Work out the finished part from the listing and answer in its coordinate system (mm). A direction names the side the tool comes from. Give positions to 0.01 mm unless a question says otherwise; leave off trailing zeros. Order: outer loops, then holes, each group sorted by start corner. A loop starts at its lowest first (then second) coordinate and runs counter-clockwise, first axis right, second up. Notation, with made-up numbers: (65.25, 1.5) -> (113.25, 1.5) arc R19 cw to (113.25, 37.5) -> close; hole circle Ø9 at (83.5, 48). An arc over 180 degrees is marked (long way). Answer as CSV lines item,"result". Start each with the question number.
1. Find the intervals of material crossed by L1, parallel to X at y = 76, z = 3.45, in increasing order.
2. A cutting plane is placed at B-B (y = 47.5). Give the vertices of the cut face in (x, z).
3. A cutting plane is placed at A-A (x = 12). Give the vertices of the cut face in (y, z).
4. For faces 4 (the flat face through (-5, 11, 3)), 5 (the flat face through (9, 79, 2)), 6 (the flat face through (0, 49, 2)), determine the directions among +Z, -Z, +X, -X, +Y, -Y from which every point of the face is accessible in a straight line to the end or side of a thin tool.
5. For a pull along X with two mould halves and no side action, classify faces 1 (the flat face through (4, 0, 3)), 2 (the flat face through (11, 45.273, 3)), 3 (the flat face through (-5, 26, 3)) as released by +X, released by -X, zero draft, split by the parting line, or undercut.
6. Flat-ended cylindrical pins translate along their axes: pin 1 (1 mm diameter, centred on y = 33, z = 3, fed in from +X); pin 2 (1.2 mm diameter, centred on x = 4, z = 2.5, fed in from +Y). Find the tip coordinate at first contact, or state that the pin passes through.
Autodesk Fusion 360 part; units mm, degrees
sketch "Sketch1" plane through (0, 0, 0) normal (0, 0, 1) x (1, 0, 0)
  line L0 (0, 0) -> (9, 0)
  line L1 (9, 0) -> (9, 83)
  line L2 (9, 83) -> (0, 83)
  line L3 (0, 83) -> (0, 0)
  dimension "d5" = 9
  dimension "d6" = 83
extrude "Extrude1" add sketch "Sketch1" along normal blind 5
sketch "Sketch2" plane through (9, 0, 0) normal (1, 0, 0) x (0, 1, 0)
  line L0 (0, 0) -> (83, 0)
  line L1 (83, 0) -> (83, 5)
  line L2 (83, 5) -> (0, 5)
  line L3 (0, 5) -> (0, 0)
  line L4 (7.5455, 5) -> (15.0909, 5)
  line L5 (15.0909, 5) -> (15.0909, 0)
  line L6 (15.0909, 0) -> (7.5455, 0)
  line L7 (7.5455, 0) -> (7.5455, 5)
  line L8 (22.6364, 0) -> (22.6364, 5)
  line L9 (22.6364, 5) -> (30.1818, 5)
  line L10 (30.1818, 0) -> (22.6364, 0)
  line L11 (30.1818, 5) -> (30.1818, 0)
  line L12 (37.7273, 0) -> (37.7273, 5)
  line L13 (37.7273, 5) -> (45.2727, 5)
  line L14 (45.2727, 0) -> (37.7273, 0)
  line L15 (45.2727, 5) -> (45.2727, 0)
  line L16 (52.8182, 0) -> (52.8182, 5)
  line L17 (52.8182, 5) -> (60.3636, 5)
  line L18 (60.3636, 0) -> (52.8182, 0)
  line L19 (60.3636, 5) -> (60.3636, 0)
  line L20 (67.9091, 0) -> (67.9091, 5)
  line L21 (67.9091, 5) -> (75.4545, 5)
  line L22 (75.4545, 0) -> (67.9091, 0)
  line L23 (75.4545, 5) -> (75.4545, 0)
  dimension "d9" = 7.5455
  dimension "d10" = 7.5455
  dimension "d13" = 60.3636
  dimension "d14" = 0
extrude "Extrude2" add sketch "Sketch2" along normal blind 5 contours L0 L2 L4 L5 L6 L7 | L0 L2 L8 L9 L10 L11 | L0 L2 L12 L13 L14 L15 | L0 L2 L16 L17 L18 L19 | L0 L2 L20 L21 L22 L23
sketch "Sketch3" plane through (0, 0, 0) normal (-1, 0, 0) x (0, -1, 0)
  line L0 (-83, 0) -> (0, 0)
  line L1 (0, 0) -> (0, 5)
  line L2 (0, 5) -> (-83, 5)
  line L3 (-83, 5) -> (-83, 0)
  line L4 (-75.4545, 5) -> (-67.9091, 5)
  line L5 (-67.9091, 5) -> (-67.9091, 0)
  line L6 (-67.9091, 0) -> (-75.4545, 0)
  line L7 (-75.4545, 0) -> (-75.4545, 5)
  line L8 (-60.3636, 0) -> (-60.3636, 5)
  line L9 (-60.3636, 5) -> (-52.8182, 5)
  line L10 (-52.8182, 0) -> (-60.3636, 0)
  line L11 (-52.8182, 5) -> (-52.8182, 0)
  line L12 (-45.2727, 0) -> (-45.2727, 5)
  line L13 (-45.2727, 5) -> (-37.7273, 5)
  line L14 (-37.7273, 0) -> (-45.2727, 0)
  line L15 (-37.7273, 5) -> (-37.7273, 0)
  line L16 (-30.1818, 0) -> (-30.1818, 5)
  line L17 (-30.1818, 5) -> (-22.6364, 5)
  line L18 (-22.6364, 0) -> (-30.1818, 0)
  line L19 (-22.6364, 5) -> (-22.6364, 0)
  line L20 (-15.0909, 0) -> (-15.0909, 5)
  line L21 (-15.0909, 5) -> (-7.5455, 5)
  line L22 (-7.5455, 0) -> (-15.0909, 0)
  line L23 (-7.5455, 5) -> (-7.5455, 0)
  point P0 (-75.4545, 5)
  dimension "d17" = 7.5455
  dimension "d20" = 60.3636
  dimension "d21" = 0
extrude "Extrude3" add sketch "Sketch3" along normal blind 5 contours L0 L2 L4 L5 L6 L7 | L0 L2 L8 L9 L10 L11 | L0 L2 L12 L13 L14 L15 | L0 L2 L16 L17 L18 L19 | L0 L2 L20 L21 L22 L23
sketch "Sketch4" plane through (0, 0, 0) normal (0, -1, 0) x (1, 0, 0)
  line L0 (0, 0) -> (9, 0)
  line L1 (9, 0) -> (9, 5)
  line L2 (9, 5) -> (0, 5)
  line L3 (0, 5) -> (0, 0)
sketch "Sketch5" plane through (0, 0, 0) normal (0, 0, 1) x (1, 0, 0)
  line L0 (-5, 0) -> (14, 0)
  line L1 (14, 0) -> (14, -5)
  line L2 (14, -5) -> (-5, -5)
  line L3 (-5, -5) -> (-5, 0)
  line L4 (0, 7.5455) -> (0, 0) construction
  line L5 (0, 0) -> (9, 0)
  point P0 (-5, 7.5455)
  dimension "d24" = 5
  dimension "d25" = 19
  dimension "d44" = 5
extrude "Extrude4" cut sketch "Sketch5" along normal blind 5
extrude "Extrude5" add sketch "Sketch5" along normal blind 5
sketch "Sketch6" plane through (0, 0, 0) normal (0, 0, 1) x (1, 0, 0)
  line L0 (-5, 83) -> (14, 83)
  line L1 (14, 83) -> (14, 88)
  line L2 (14, 88) -> (-5, 88)
  line L3 (-5, 88) -> (-5, 83)
  line L4 (9, 83) -> (0, 83)
  point P0 (0, 83)
  point P1 (-5, 75.4545)
  dimension "d31" = 19
  dimension "d32" = 5
  dimension "d43" = 5
extrude "Extrude6" cut sketch "Sketch6" along normal blind 5
extrude "Extrude7" add sketch "Sketch6" along normal blind 5
sketch "Sketch7" plane through (0, 0, 5) normal (0, 0, 1) x (-1, 0, 0)
  line L0 (0, -83) -> (0, -75.4545)
  line L1 (0, -75.4545) -> (5, -75.4545)
  line L2 (5, -75.4545) -> (5, -67.9091)
  line L3 (5, -67.9091) -> (0, -67.9091)
  line L4 (0, -67.9091) -> (0, -60.3636)
  line L5 (0, -60.3636) -> (5, -60.3636)
  line L6 (5, -60.3636) -> (5, -52.8182)
  line L7 (5, -52.8182) -> (0, -52.8182)
  line L8 (0, -52.8182) -> (0, -45.2727)
  line L9 (0, -45.2727) -> (5, -45.2727)
  line L10 (5, -45.2727) -> (5, -37.7273)
  line L11 (5, -37.7273) -> (0, -37.7273)
  line L12 (0, -37.7273) -> (0, -30.1818)
  line L13 (0, -30.1818) -> (5, -30.1818)
  line L14 (5, -30.1818) -> (5, -22.6364)
  line L15 (5, -22.6364) -> (0, -22.6364)
  line L16 (0, -22.6364) -> (0, -15.0909)
  line L17 (0, -15.0909) -> (5, -15.0909)
  line L18 (5, -15.0909) -> (5, -7.5455)
  line L19 (5, -7.5455) -> (0, -7.5455)
  line L20 (0, -7.5455) -> (0, 0)
  line L21 (0, 0) -> (5, 0)
  line L22 (5, 0) -> (5, 5)
  line L23 (5, 5) -> (-14, 5)
  line L24 (-14, 5) -> (-14, 0)
  line L25 (-14, 0) -> (-9, 0)
  line L26 (-9, 0) -> (-9, -7.5455)
  line L27 (-9, -7.5455) -> (-14, -7.5455)
  line L28 (-14, -7.5455) -> (-14, -15.0909)
  line L29 (-14, -15.0909) -> (-9, -15.0909)
  line L30 (-9, -15.0909) -> (-9, -22.6364)
  line L31 (-9, -22.6364) -> (-14, -22.6364)
  line L32 (-14, -22.6364) -> (-14, -30.1818)
  line L33 (-14, -30.1818) -> (-9, -30.1818)
  line L34 (-9, -30.1818) -> (-9, -37.7273)
  line L35 (-9, -37.7273) -> (-14, -37.7273)
  line L36 (-14, -37.7273) -> (-14, -45.2727)
  line L37 (-14, -45.2727) -> (-9, -45.2727)
  line L38 (-9, -45.2727) -> (-9, -52.8182)
  line L39 (-9, -52.8182) -> (-14, -52.8182)
  line L40 (-14, -52.8182) -> (-14, -60.3636)
  line L41 (-14, -60.3636) -> (-9, -60.3636)
  line L42 (-9, -60.3636) -> (-9, -67.9091)
  line L43 (-9, -67.9091) -> (-14, -67.9091)
  line L44 (-14, -67.9091) -> (-14, -75.4545)
  line L45 (-14, -75.4545) -> (-9, -75.4545)
  line L46 (-9, -75.4545) -> (-9, -83)
  line L47 (-9, -83) -> (-14, -83)
  line L48 (-14, -83) -> (-14, -88)
  line L49 (-14, -88) -> (5, -88)
  line L50 (5, -88) -> (5, -83)
  line L51 (5, -83) -> (0, -83)
  line L52 (-2.5, 0) -> (-6.5, 0)
  line L53 (-6.5, 0) -> (-6.5, 5)
  line L54 (-6.5, 5) -> (-2.5, 5)
  line L55 (-2.5, 5) -> (-2.5, 0)
  line L56 (-6.5, 0) -> (-9, 0) construction
  line L57 (0, 0) -> (-2.5, 0) construction
  line L58 (-2.5, -88) -> (-6.5, -88)
  line L59 (-6.5, -88) -> (-6.5, -83)
  line L60 (-6.5, -83) -> (-2.5, -83)
  line L61 (-2.5, -83) -> (-2.5, -88)
  line L62 (-6.5, -83) -> (-9, -83) construction
  line L63 (-2.5, -83) -> (0, -83) construction
  dimension "d41" = 4
  dimension "d42" = 5
  dimension "d45" = 5
  dimension "d46" = 4
extrude "Extrude9" cut sketch "Sketch7" against normal blind 5 contours L23 L52 L53 L54 L55
extrude "Extrude8" cut sketch "Sketch7" against normal blind 5 contours L49 L58 L59 L60 L61
equation "paksus = 5 mm"
equation "pikkus = 83 mm"
equation "pikkus_tapp = pikkus / 11"
equation "laius = 9 mm"
equation "d5 = laius"
equation "d6 = pikkus"
equation "d7 = paksus"
equation "d9 = pikkus_tapp"
equation "d10 = pikkus_tapp"
equation "d13 = pikkus - 2 * pikkus_tapp - pikkus_tapp"
equation "d15 = paksus"
equation "d17 = pikkus_tapp"
equation "d20 = pikkus - 2 * pikkus_tapp - pikkus_tapp"
equation "d22 = paksus"
equation "d24 = paksus"
equation "d25 = 2 * paksus + laius"
equation "d27 = paksus"
equation "d29 = paksus"
equation "d31 = 2 * paksus + laius"
equation "d32 = paksus"
equation "d34 = paksus"
equation "d36 = paksus"
equation "d44 = paksus"
equation "d45 = paksus"
Answer sheet:
1,L1,"x = 0 to 9"
2,outline,"(0, 0) -> (9, 0) -> (9, 5) -> (0, 5) -> close"
3,outline,"(-5, 0) -> (0, 0) -> (0, 5) -> (-5, 5) -> close; (7.55, 0) -> (15.09, 0) -> (15.09, 5) -> (7.55, 5) -> close; (22.64, 0) -> (30.18, 0) -> (30.18, 5) -> (22.64, 5) -> close; (37.73, 0) -> (45.27, 0) -> (45.27, 5) -> (37.73, 5) -> close; (52.82, 0) -> (60.36, 0) -> (60.36, 5) -> (52.82, 5) -> close; (67.91, 0) -> (75.45, 0) -> (75.45, 5) -> (67.91, 5) -> close; (83, 0) -> (88, 0) -> (88, 5) -> (83, 5) -> close"
4,face 4,"+Z, -Z, -X, +Y, -Y"
4,face 5,"+Z, -Z, +X"
4,face 6,"+Z, -Z, -X"
5,face 1,"undercut"
5,face 2,"zero draft"
5,face 3,"released by -X"
6,pin 1,"stops at x = 9"
6,pin 2,"stops at y = 83"
